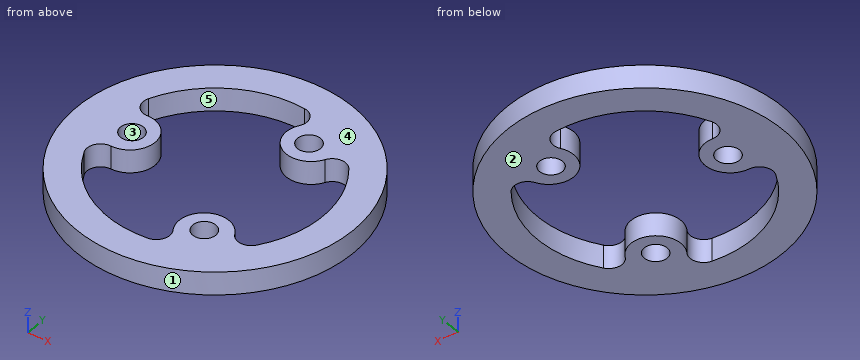
from build123d import *

# Parameters (mm, degrees)
ESQUISSE1_R        = 18
ESQUISSE1_R_2      = 1.5
BOSS_EXTRU_1_DEPTH = 3


with BuildPart() as part:
    # Esquisse1 → Boss.-Extru.1 (new body)
    with BuildSketch(Plane.XY):
        Circle(ESQUISSE1_R)
        with Locations((5.240453276, 9.386167986)):
            Circle(ESQUISSE1_R_2, mode=Mode.SUBTRACT)
        with Locations((5.508433282, -9.231449657)):
            Circle(ESQUISSE1_R_2, mode=Mode.SUBTRACT)
        with Locations((-10.748886558, -0.154718329)):
            Circle(ESQUISSE1_R_2, mode=Mode.SUBTRACT)
        with BuildLine():
            ThreePointArc((11.453630047, -8.050736534), (13.998549936, 0.201493638), (11.217170127, 8.377057619))
            ThreePointArc((11.217170127, 8.377057619), (9.667160345, 9.073667479), (8.256579008, 8.126009358))
            ThreePointArc((8.256579008, 8.126009358), (3.778001199, 6.766772269), (2.58509342, 11.292493835))
            ThreePointArc((2.58509342, 11.292493835), (2.651653429, 12.990541357), (1.245327334, 13.944502853))
            ThreePointArc((1.245327334, 13.944502853), (-7.173773577, 12.022353042), (-12.86332977, 5.525825479))
            ThreePointArc((-12.86332977, 5.525825479), (-12.691606715, 3.835172702), (-11.165620039, 3.087402491))
            ThreePointArc((-11.165620039, 3.087402491), (-7.749197286, -0.111541121), (-11.072133243, -3.407490345))
            ThreePointArc((-11.072133243, -3.407490345), (-12.575965538, -4.198871447), (-12.698957381, -5.893766319))
            ThreePointArc((-12.698957381, -5.893766319), (-6.824776359, -12.22384668), (1.646159643, -13.902883098))
            ThreePointArc((1.646159643, -13.902883098), (3.02444637, -12.90884018), (2.909041031, -11.213411848))
            ThreePointArc((2.909041031, -11.213411848), (3.971196087, -6.655231148), (8.487039823, -7.88500349))
            ThreePointArc((8.487039823, -7.88500349), (9.92431211, -8.79166991), (11.453630047, -8.050736534))
        make_face(mode=Mode.SUBTRACT)
    extrude(amount=BOSS_EXTRU_1_DEPTH)


solid = part.part
Check sheet for the modelled part. Datum: model origin and axes. Units: mm. Face numbers are marked on the shaded views. A direction names the side the tool comes from. Give positions to 0.01 mm unless a question says otherwise; leave off trailing zeros. Write each loop counter-clockwise with the first axis right and the second up, starting at its lowest first coordinate (ties: lowest second). Pieces come first, ordered by that corner, then holes. Notation, with made-up numbers: (9.25, 11) -> (17.25, 11) arc R25 cw to (17.25, 27) -> close; hole circle Ø11 at (75, 23). An arc over 180 degrees is marked (long way). One line per item, written item: value. Start each with the question number.
Item 1: Draft check along X on the marked faces 1, 2 and 3. Enter one of: +X half, -X half, draft (parallel to the pull), parting line (faces both ways), or undercut.
Item 2: Section check B-B on y = 0.5. Record the cut outline in (x, z).
Item 3: Section check C-C on z = 1.35. State how many separate pieces and enclosed holes the cut face has, then the cut area to 3 significant figures.
Item 4: Section check D-D on y = -12.5. Record the cut outline in (x, z), then the cut area to 3 significant figures.
Item 5: Gauge pin test, flat end, axial feed: pin 1 (2.5 mm diameter, centred on x = 5.51, y = -9.23, fed in from +Z). Record the tip position at first contact, or that the pin passes through.
Item 6: Material ranges on probe 1 along Y at (x, z) = (0, 2.3); probe 2 along Y at (x, z) = (-8.5, 2.8); probe 3 along Y at (x, z) = (3, 1.55), recorded low to high. Write a range as from..to.
Item 7: Section check A-A on x = 0. Record the cut outline in (y, z), then the cut area to 3 significant figures.
Item 8: Tool access check on the marked faces 4 and 5. Record the directions out of +Z, -Z, +X, -X, +Y, -Y that give a thin tool (end or side, any length) a straight path to the whole face; none if there is none.
Results list:
1. face 1: parting line
1. face 2: draft
1. face 3: undercut
2. outline: (-17.99, 0) -> (-12.1, 0) -> (-12.1, 3) -> (-17.99, 3) -> close; (-9.4, 0) -> (-7.82, 0) -> (-7.82, 3) -> (-9.4, 3) -> close; (13.99, 0) -> (17.99, 0) -> (17.99, 3) -> (13.99, 3) -> close
3. separate pieces: 1
3. enclosed holes: 4
3. area: 495 mm²
4. outline: (-12.95, 0) -> (-6.3, 0) -> (-6.3, 3) -> (-12.95, 3) -> close; (3.16, 0) -> (12.95, 0) -> (12.95, 3) -> (3.16, 3) -> close
4. area: 49.3 mm²
5. pin 1: through
6. probe 1: -18..-14, 14..18
6. probe 2: -15.87..-11.12, -2.24..1.92, 11.12..15.87
6. probe 3: -17.75..-12.96, -11.37..-7.55, 7.37..17.75
7. outline: (-18, 0) -> (-14, 0) -> (-14, 3) -> (-18, 3) -> close; (14, 0) -> (18, 0) -> (18, 3) -> (14, 3) -> close
7. area: 24.0 mm²
8. face 4: +Z, +X, -X, +Y, -Y
8. face 5: +Z, -Z
